from build123d import *

# Parameters (mm, degrees)
F1_DEPTH  = 16
F2_W      = 44
F2_H      = 30
F3_DEPTH  = 18
F4_R      = 8
F5_DEPTH  = 22
F7_DEPTH  = 26
F9_DEPTH  = 42
F11_DEPTH = 20.001
F13_DEPTH = 20


with BuildPart() as f1:
    # F0 (on Front) → F1 (new body)
    with BuildSketch(Plane.XZ):
        Polygon((0, 40), (0, 0), (10, 0), (10, -6), (34, -6), (34, 0), (44, 0), (44, 40), align=None)
    extrude(amount=F1_DEPTH)

    # F2 (on face) → F3 (join)
    with BuildSketch(Plane.XZ):
        Polygon((0, 52), (0, 40), (44, 40), (44, 10), (120, 10), (120, 26.019238), (75, 52), align=None)
        with Locations((22, 25)):
            Rectangle(F2_W, F2_H)
    extrude(amount=-F3_DEPTH)

    # F4 (on face) → F5 (cut)
    with BuildSketch(Plane.XZ.offset(16)):
        with Locations((22, 22)):
            Circle(F4_R)
    extrude(amount=-F5_DEPTH, mode=Mode.SUBTRACT)

    # F6 (on face) → F7 (join)
    with BuildSketch(Plane.XZ):
        Polygon((44, 10), (0, 10), (0, 0), (10, 0), (10, -6), (34, -6), (34, 0), (44, 0), align=None)
    extrude(amount=-F7_DEPTH)

    # F8 (on face) → F9 (join)
    with BuildSketch(Plane(origin=(0, 0, 10), x_dir=(1, 0, 0), z_dir=(0, 0, -1))):
        Polygon((85.358984, -18), (85.358984, -38), (120, -18), align=None)
    extrude(amount=-F9_DEPTH)

    # F10 (on face) → F11 (cut, through all)
    with BuildSketch(Plane.XZ.offset(-18)):
        Polygon((120, 52), (85.358984, 52), (85.358984, 46.019238), (120, 26.019238), align=None)
    extrude(amount=-F11_DEPTH, mode=Mode.SUBTRACT)

    # F12 (on face) → F13 (join)
    with BuildSketch(Plane(origin=(0, 18, 0), x_dir=(-1, 0, 0), z_dir=(0, 1, 0))):
        Polygon((-75, 52), (-85.358984, 46.019238), (-85.358984, 10), (-44, 10), (0, 10), (0, 52), align=None)
    extrude(amount=F13_DEPTH)


solid = f1.part
Verification items for the finished model (mm, model axes). A direction names the side the tool comes from. Give positions to 0.01 mm unless a question says otherwise; leave off trailing zeros. Write each loop counter-clockwise with the first axis right and the second up, starting at its lowest first coordinate (ties: lowest second). Pieces come first, ordered by that corner, then holes.
(1) Cross-section at C-C (x = 22). Enter the section's corners in (y, z).
(2) Gauge pin test, flat ends, axial feed: pin 1 (21 mm diameter, centred on x = 66, z = 34.5, fed in from -Y); pin 2 (3 mm diameter, centred on x = 3.5, y = -5.5, fed in from -Z); pin 3 (12 mm diameter, centred on y = 24.5, z = 10.5, fed in from +X). Record the tip position at first contact, or that the pin passes through.
(3) Cross-section at B-B (z = 22). Enter the section's corners in (x, y), plus the area to 3 significant figures.
(4) Material ranges on line 1 (Z direction, x = 22, y = -5.75); line 2 (Z direction, x = 22, y = 1); line 3 (X direction, y = 5, z = -1), recorded low to high.
(5) Access from +Z, -Z, +X, -X, +Y, -Y to the whole of each face (thin tool, end or side, straight path). Record for faces 1 (the face through (39, 5, 0)), 2 (the face through (5, 5, 0)), 3 (the face through (22, -8, 40)), 4 (the face through (22, 26, 4)).
(6) Cross-section at A-A (y = 12). Enter the section's corners in (x, z), plus the area to 3 significant figures.
(7) Cross-section at D-D (y = -7). Enter the section's corners in (x, z), plus the area to 3 significant figures.
(8) Mould release check, pull along Z, two halves, no side actions. Record for faces 5 (the face through (37, 19, 52)), 6 (the face through (16.1, -5.2, 27.4)), 7 (the face through (59, 0, 31)), 8 (the face through (22, 5, -6)): +Z half, -Z half, draft (parallel to the pull), parting line (faces both ways), or undercut.
Worked out:
1. outline: (-16, -6) - (26, -6) - (26, 10) - (38, 10) - (38, 52) - (0, 52) - (0, 40) - (-16, 40) - (-16, 30) - (6, 30) - (6, 14) - (-16, 14) - close
2. pin 1: stops at y = 0
2. pin 2: stops at z = 0
2. pin 3: stops at x = 119.13
3. outline: (0, -16) - (14, -16) - (14, 6) - (30, 6) - (30, -16) - (44, -16) - (44, 0) - (120, 0) - (120, 18) - (85.36, 38) - (0, 38) - close
3. area: 4,570 mm2
4. line 1: z = -6 to 14, 30 to 40
4. line 2: z = -6 to 14, 30 to 52
4. line 3: x = 10 to 34
5. face 1: -Z, +X, +Y, -Y
5. face 2: -Z, -X, +Y, -Y
5. face 3: +Z, +X, -X, -Y
5. face 4: -Z, +X, -X, +Y
6. outline: (0, 0) - (10, 0) - (10, -6) - (34, -6) - (34, 0) - (44, 0) - (44, 10) - (120, 10) - (120, 26.02) - (75, 52) - (0, 52) - close
6. area: 5,040 mm2
7. outline: (0, 0) - (10, 0) - (10, -6) - (34, -6) - (34, 0) - (44, 0) - (44, 40) - (0, 40) - close; hole circle Ø16 at (22, 22)
7. area: 1,700 mm2
8. face 5: +Z half
8. face 6: undercut
8. face 7: draft
8. face 8: -Z half
